from build123d import *

# Parameters (mm, degrees)
SKIZZE1_W                            = 40.7
SKIZZE1_H                            = 35.7
AUFSATZ_LINEAR_AUSTRAGEN1_DEPTH      = 20.2
AUFSATZ_LINEAR_AUSTRAGEN2_DEPTH      = 8
AUFSATZ_LINEAR_AUSTRAGEN2_DEPTH_BACK = 48.7
SKIZZE2_W                            = 18
SKIZZE2_H                            = 2.5
SKIZZE3_R                            = 2.25
SCHNITT_LINEAR_AUSTRAGEN1_DEPTH      = 8
SKIZZE4_R                            = 7
AUFSATZ_LINEAR_AUSTRAGEN3_DEPTH      = 1.5
SKIZZE5_R                            = 3
AUFSATZ_LINEAR_AUSTRAGEN4_DEPTH      = 4
SKIZZE6_W                            = 6
SKIZZE6_H                            = 3.5
AUFSATZ_LINEAR_AUSTRAGEN5_DEPTH      = 4


with BuildPart() as part:
    # Skizze1 → Aufsatz-Linear austragen1 (new body)
    with BuildSketch(Plane.XY):
        with Locations((20.35, 17.85)):
            Rectangle(SKIZZE1_W, SKIZZE1_H)
    extrude(amount=AUFSATZ_LINEAR_AUSTRAGEN1_DEPTH)

    # Skizze2 → Aufsatz-Linear austragen2 (add, two sides: drawn at the far end of the back side and taken through both)
    with BuildSketch(Plane(origin=(40.7, 0, 0), x_dir=(0, 0, -1), z_dir=(1, 0, 0)).offset(-AUFSATZ_LINEAR_AUSTRAGEN2_DEPTH_BACK)):
        with Locations((-10.1, 27.25)):
            Rectangle(SKIZZE2_W, SKIZZE2_H)
    extrude(amount=AUFSATZ_LINEAR_AUSTRAGEN2_DEPTH + AUFSATZ_LINEAR_AUSTRAGEN2_DEPTH_BACK)

    # Skizze3 → Schnitt-Linear austragen1 (cut)
    with BuildSketch(Plane(origin=(0, 28.5, 0), x_dir=(1, 0, 0), z_dir=(0, 1, 0))):
        with Locations(Location((45.15, -5.25, 0), (0, 0, 180))):
            Circle(SKIZZE3_R)
        with Locations(Location((45.15, -14.95, 0), (0, 0, 180))):
            Circle(SKIZZE3_R)
        with Locations(Location((-4.45, -5.25, 0), (0, 0, 180))):
            Circle(SKIZZE3_R)
        with Locations(Location((-4.45, -14.95, 0), (0, 0, 180))):
            Circle(SKIZZE3_R)
    extrude(amount=-SCHNITT_LINEAR_AUSTRAGEN1_DEPTH, mode=Mode.SUBTRACT)

    # Skizze4 → Aufsatz-Linear austragen3 (add)
    with BuildSketch(Plane(origin=(0, 35.7, 0), x_dir=(1, 0, 0), z_dir=(0, 1, 0))):
        with Locations(Location((8.5, -10.1, 0), (0, 0, 90))):
            Circle(SKIZZE4_R)
    extrude(amount=AUFSATZ_LINEAR_AUSTRAGEN3_DEPTH)

    # Skizze5 → Aufsatz-Linear austragen4 (add)
    with BuildSketch(Plane(origin=(0, 37.2, 0), x_dir=(1, 0, 0), z_dir=(0, 1, 0))):
        with Locations(Location((8.5, -10.1, 0), (0, 0, 270))):
            Circle(SKIZZE5_R)
    extrude(amount=AUFSATZ_LINEAR_AUSTRAGEN4_DEPTH)

    # Skizze6 → Aufsatz-Linear austragen5 (add)
    with BuildSketch(Plane.ZY):
        with Locations((10.1, 2.75)):
            Rectangle(SKIZZE6_W, SKIZZE6_H)
    extrude(amount=AUFSATZ_LINEAR_AUSTRAGEN5_DEPTH)


solid = part.part
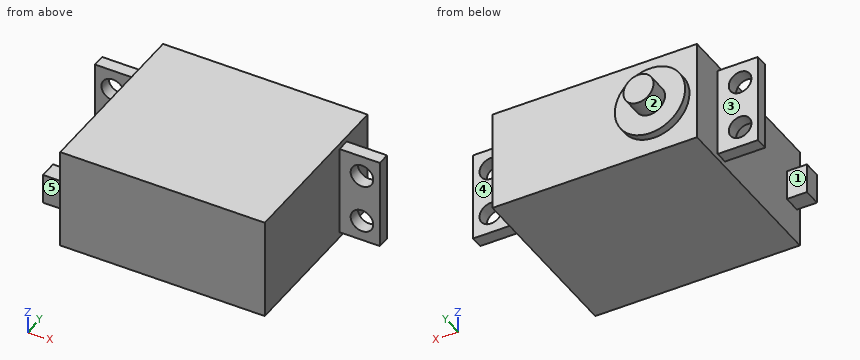
The model under review builds one solid part; all positions refer to its coordinate system, in mm. Face numbers are marked on the shaded views. A direction names the side the tool comes from. Coordinates: 2 decimals unless noted, no trailing zeros. Loops run counter-clockwise (first coordinate to the right, second up) from the corner with the lowest first, then second, coordinate; pieces in that order, holes last. Notation, with made-up numbers: (-16.5, -8) -> (40.5, -8) arc R15 ccw to (40.5, 16) -> close; hole circle Ø8 at (-30.5, -23.75). An arc over 180 degrees is marked (long way). Use a Markdown table: item, result. Add a question column.
1. Machinability: for the marked faces 1, 2, 3, 4 and 5, which of the approach directions +Z, -Z, +X, -X, +Y, -Y give a long, thin tool a straight path to every point of the face, cutting with its end or side? Answer none if there is none.
2. Add section D-D on y = 23.5. Write out the cut boundary in (x, z), plus the area to 3 significant figures.
3. To check wall thickness, follow line 1 (Z direction, x = 45, y = 27) (3 decimals); line 2 (Y direction, x = 10, z = 4.25); line 3 (Y direction, x = 27, z = 16). State the ranges of each line that lie inside material, in increasing order.
4. Clearance check with flat-ended pins moving along their axes: pin 1 Ø10 at (x, z) = (16, 8) entering from +Y; pin 2 Ø1 at (x, y) = (-1.5, 3.5) entering from -Z; pin 3 Ø5 at (x, z) = (4.5, 6) entering from +Y; pin 4 Ø6.5 at (x, z) = (-5.5, 8.5) entering from -Y. State where each tip first meets the part, or that it passes through.
5. Add section A-A on x = 8.5. Write out the cut boundary in (y, z).
6. Add section C-C on z = 5.25. Write out the cut boundary in (x, y), plus the area to 3 significant figures.
7. Add section B-B on z = 2. Write out the cut boundary in (x, y), plus the area to 3 significant figures.
Returned:
| question | item | result |
|---|---|---|
| 1 | face 1 | +Z, -Z, -X |
| 1 | face 2 | +Y |
| 1 | face 3 | +Z, -Z, -X, +Y |
| 1 | face 4 | +Z, -Z, +X, +Y |
| 1 | face 5 | +Z, -Z, -X, -Y |
| 2 | outline | (0, 0) -> (40.7, 0) -> (40.7, 20.2) -> (0, 20.2) -> close |
| 2 | area | 822 mm² |
| 3 | line 1 | z = 1.1 to 3.005, 7.495 to 12.705, 17.195 to 19.1 |
| 3 | line 2 | y = 0 to 37.2 |
| 3 | line 3 | y = 0 to 35.7 |
| 4 | pin 1 | stops at y = 41.2 |
| 4 | pin 2 | stops at z = 7.1 |
| 4 | pin 3 | stops at y = 37.2 |
| 4 | pin 4 | stops at y = 1 |
| 5 | outline | (0, 0) -> (35.7, 0) -> (35.7, 3.1) -> (37.2, 3.1) -> (37.2, 7.1) -> (41.2, 7.1) -> (41.2, 13.1) -> (37.2, 13.1) -> (37.2, 17.1) -> (35.7, 17.1) -> (35.7, 20.2) -> (0, 20.2) -> close |
| 6 | outline | (-8, 26) -> (-6.7, 26) -> (-6.7, 28.5) -> (-8, 28.5) -> close; (-2.2, 26) -> (0, 26) -> (0, 0) -> (40.7, 0) -> (40.7, 26) -> (42.9, 26) -> (42.9, 28.5) -> (40.7, 28.5) -> (40.7, 35.7) -> (13.55, 35.7) -> (13.55, 37.2) -> (3.45, 37.2) -> (3.45, 35.7) -> (0, 35.7) -> (0, 28.5) -> (-2.2, 28.5) -> close; (47.4, 26) -> (48.7, 26) -> (48.7, 28.5) -> (47.4, 28.5) -> close |
| 6 | area | 1,490 mm² |
| 7 | outline | (-8, 26) -> (0, 26) -> (0, 0) -> (40.7, 0) -> (40.7, 26) -> (48.7, 26) -> (48.7, 28.5) -> (40.7, 28.5) -> (40.7, 35.7) -> (0, 35.7) -> (0, 28.5) -> (-8, 28.5) -> close |
| 7 | area | 1,490 mm² |
